Part model, mm, in its own coordinate system. A direction names the side the tool comes from. Round coordinates to 2 decimals unless told otherwise and drop trailing zeros. Order: outer loops, then holes, each group sorted by start corner. A loop starts at its lowest first (then second) coordinate and runs counter-clockwise, first axis right, second up. Notation, with made-up numbers: M 61.5,-35.5 L 92.5,-35.5 A14 ccw 92.5,-27.5 Z; hole C -2,77.5 d8. An arc over 180 degrees is marked long. Write each question's results on one line, items separated by ' | '. Start each with the question number.
1. Band-saw the part on D-D, the plane y = 12. List the corners of the cut face in (x, z) (3 decimals).
2. Two-plate mould, pull along X, no slides. Class faces 1 (the face through (19.05, 0, 0)), 2 (the face through (-3, -15.875, 0)), 3 (the face through (1.34, -17.48, -10.6)), 4 (the face through (-18.573, -16.328, 0.267)): +X half, -X half, draft (parallel to the pull), parting line (faces both ways), or undercut.
3. Band-saw the part on A-A, the plane x = 0. List the corners of the cut face in (y, z) (3 decimals).
4. Band-saw the part on B-B, the plane z = -12.7. Give the number of separate pieces and of enclosed holes in the cut face, then the cut area to 3 significant figures.
5. Which spindle directions (+Z, -Z, +X, -X, +Y, -Y) get a long thin tool onto all of the face, cutting with end or side? Do faces 5 (the face through (15.875, 3, 0)), 6 (the face through (8, -17, -19.05)). Say none if no direction does.
6. Drop a flat-ended pin along its axis: pin 1 Ø14.5 at (x, z) = (-5.5, 1.5) entering from +Y (3 decimals). Give the stop position or say it passes through.
7. Probe L1, parallel to Z at x = 0, y = -18.1; L2, parallel to X at y = 2, z = -2.5 (3 decimals); L3, parallel to Y at x = -5, z = 9 (3 decimals). List the from-to ranges inside material, lowest first. Write a range as [from, to].
```python
from build123d import *

# Parameters (mm, degrees)
BOSS_EXTRUDE1_DEPTH = 19.05
SKETCH3_R           = 2.4892
CUT_EXTRUDE1_DEPTH  = 47.6627796
SKETCH4_R           = 2.4892
CUT_EXTRUDE2_DEPTH  = 47.6627796


with BuildPart() as part:
    # Sketch2 → Boss-Extrude1 (new, symmetric)
    with BuildSketch(Plane.XY):
        with BuildLine():
            Line((-19.05, -19.05), (19.05, -19.05))
            Line((19.05, -19.05), (19.05, 19.05))
            Line((19.05, 19.05), (17.4625, 19.05))
            ThreePointArc((17.4625, 19.05), (16.339967985, 18.585032015), (15.875, 17.4625))
            Line((15.875, 17.4625), (15.875, -11.0998))
            ThreePointArc((15.875, -11.0998), (14.476376302, -14.476376302), (11.0998, -15.875))
            Line((11.0998, -15.875), (-17.4625, -15.875))
            ThreePointArc((-17.4625, -15.875), (-18.585032015, -16.339967985), (-19.05, -17.4625))
            Line((-19.05, -17.4625), (-19.05, -19.05))
        make_face()
    extrude(amount=BOSS_EXTRUDE1_DEPTH, both=True)

    # Sketch3 → Cut-Extrude1 (cut, through all)
    with BuildSketch(Plane(origin=(19.05, 0, 0), x_dir=(0, 0, -1), z_dir=(1, 0, 0))):
        with Locations(Location((-12.7, 3.96875, 0), (0, 0, 90))):
            Circle(SKETCH3_R)
        with Locations(Location((12.7, 3.96875, 0), (0, 0, 90))):
            Circle(SKETCH3_R)
    extrude(amount=-CUT_EXTRUDE1_DEPTH, mode=Mode.SUBTRACT)

    # Sketch4 → Cut-Extrude2 (cut, through all)
    with BuildSketch(Plane.XZ.offset(19.05)):
        with Locations((0, 12.7)):
            Circle(SKETCH4_R)
        with Locations((0, -12.7)):
            Circle(SKETCH4_R)
    extrude(amount=-CUT_EXTRUDE2_DEPTH, mode=Mode.SUBTRACT)


solid = part.part
```
Solution:
1) outline: M 15.875,-19.05 L 19.05,-19.05 L 19.05,19.05 L 15.875,19.05 Z
2) face 1: +X half | face 2: draft | face 3: undercut | face 4: -X half
3) outline: M -19.05,-19.05 L -15.875,-19.05 L -15.875,-15.189 L -19.05,-15.189 Z; M -19.05,-10.211 L -15.875,-10.211 L -15.875,10.211 L -19.05,10.211 Z; M -19.05,15.189 L -15.875,15.189 L -15.875,19.05 L -19.05,19.05 Z
4) separate pieces: 3 | enclosed holes: 0 | area: 204 mm^2
5) face 5: +Z, -Z, -X, +Y | face 6: -Z, +X, -X, +Y, -Y
6) pin 1: y = -15.875
7) L1: [-19.05, -15.19], [-10.21, 10.21], [15.19, 19.05] | L2: [15.875, 19.05] | L3: [-19.05, -15.875]
